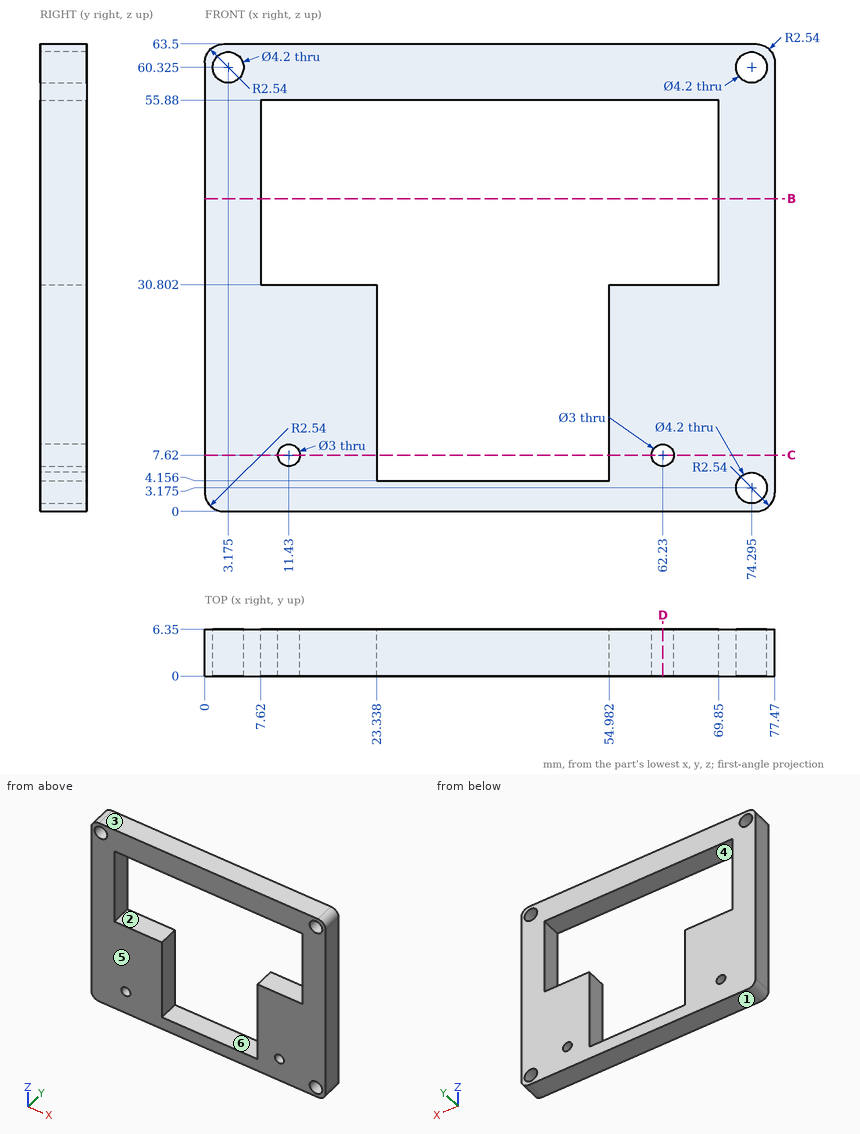
Geometry check sheet. Reference: drawing and pictorial views, mm from the part's lowest x, y, z. A direction names the side the tool comes from. Round coordinates to 2 decimals unless told otherwise and drop trailing zeros. Loops run counter-clockwise (first coordinate to the right, second up) from the corner with the lowest first, then second, coordinate; pieces in that order, holes last. Notation, with made-up numbers: (-1.75, 61) -> (50.25, 61) arc R6 cw to (50.25, 65) -> close; hole circle Ø11 at (-16, -20.5). An arc over 180 degrees is marked (long way). Answer as a JSON object with one key per item and string values. Group by question number.
Item 1: Set-up check for the marked faces 1 and 2: record each of +Z, -Z, +X, -X, +Y, -Y from which the full face is reachable in a straight line by a thin tool's end or side.
Item 2: Depth check by flat-ended pin: pin 1 Ø2.5 at (x, z) = (11.43, 7.62) entering from -Y. Enter the tip coordinate at first touch or a pass-through.
Item 3: Cross-section at C-C, the plane z = 7.62. Record the cut outline in (x, y).
Item 4: Cross-section at B-B, the plane z = 42.5. Record the cut outline in (x, y).
Item 5: Cross-section at D-D, the plane x = 62.23. Record the cut outline in (y, z).
Item 6: Thickness scan on line 1 along Z through (x, y) = (34.5, 3) (1 decimal); line 2 along X through (y, z) = (4, 43); line 3 along Z through (x, y) = (74, 3.25) (1 decimal). Record the ranges inside material, lowest first.
Item 7: Release check for a two-part mould opening along Z. For the marked faces 3, 4, 5 and 6 record: pulls with the +Z half, pulls with the -Z half, needs draft (parallel to the pull), parting line crosses it, or undercut.
Determined:
{
 "1": {"face 1": "-Z, +X, -X, +Y, -Y", "face 2": "+Y, -Y"},
 "2": {"pin 1": "passes through"},
 "3": {"outline": "(0, 0) -> (9.93, 0) -> (9.93, 6.35) -> (0, 6.35) -> close; (12.93, 0) -> (23.34, 0) -> (23.34, 6.35) -> (12.93, 6.35) -> close; (54.98, 0) -> (60.73, 0) -> (60.73, 6.35) -> (54.98, 6.35) -> close; (63.73, 0) -> (77.47, 0) -> (77.47, 6.35) -> (63.73, 6.35) -> close"},
 "4": {"outline": "(0, 0) -> (7.62, 0) -> (7.62, 6.35) -> (0, 6.35) -> close; (69.85, 0) -> (77.47, 0) -> (77.47, 6.35) -> (69.85, 6.35) -> close"},
 "5": {"outline": "(0, 0) -> (6.35, 0) -> (6.35, 6.12) -> (0, 6.12) -> close; (0, 9.12) -> (6.35, 9.12) -> (6.35, 30.8) -> (0, 30.8) -> close; (0, 55.88) -> (6.35, 55.88) -> (6.35, 63.5) -> (0, 63.5) -> close"},
 "6": {"line 1": "z = 0 to 4.2, 55.9 to 63.5", "line 2": "x = 0 to 7.62, 69.85 to 77.47", "line 3": "z = 0 to 1.1, 5.3 to 58.2, 62.4 to 63.5"},
 "7": {"face 3": "pulls with the +Z half", "face 4": "undercut", "face 5": "needs draft", "face 6": "undercut"}
}
